from build123d import *


with BuildPart() as part:
    # Sketch2 → Revolve1 (revolve)
    with BuildSketch(Plane.XY, mode=Mode.PRIVATE) as revolve1_sk:
        with BuildLine():
            Line((0, 0), (6.24, 0))
            Line((6.24, 0), (6.24, 48.588483168))
            ThreePointArc((6.24, 48.588483168), (6.146561159, 49.109622023), (5.877885725, 49.565834731))
            ThreePointArc((5.877885725, 49.565834731), (4.874570596, 52.273796489), (5.877885725, 54.981758248))
            ThreePointArc((5.877885725, 54.981758248), (6.146561159, 55.437970955), (6.24, 55.95910981))
            Line((6.24, 55.95910981), (6.24, 55.998530254))
            ThreePointArc((6.24, 55.998530254), (4.278763618, 60.161301491), (0, 61.854610207))
            Line((0, 61.854610207), (0, 0))
        make_face()
    revolve(revolve1_sk.sketch.rotate(Axis((0, 61.854610207, 0), (0, -1, 0)), 180), axis=Axis((0, 61.854610207, 0), (0, -1, 0)))


solid = part.part
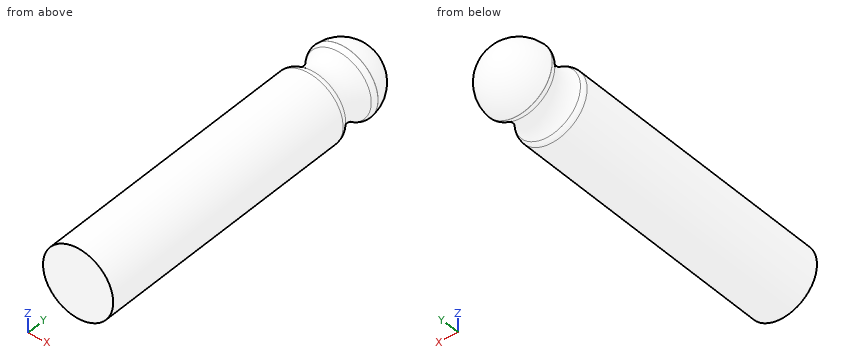
Could you check a few things on this model? Use its own coordinates, in mm. Give positions to 0.01 mm unless a question says otherwise; leave off trailing zeros. Write each loop counter-clockwise with the first axis right and the second up, starting at its lowest first coordinate (ties: lowest second). Pieces come first, ordered by that corner, then holes. Notation, with made-up numbers: (12.25, -16.75) -> (29.25, -16.75) arc R17 ccw to (29.25, -11.75) -> close; hole circle Ø10 at (-9, -28.5). An arc over 180 degrees is marked (long way). Answer as a JSON object with one key per item and string values.
Q1. Suppose I cut it at D-D on y = 51. Write out the boundary of the cut face in (x, z).
Taken from the geometry:
{"outline": "circle Ø10.15 at (0, 0)"}
Q2. Please list where these lines run through material, in increasing order: L1, parallel to X at y = 12.5, z = -0.25; L2, parallel to X at y = 25, z = -2.5; L3, parallel to Y at x = 4.25, z = -0.75.
Taken from the geometry:
{"L1": "x = -6.23 to 6.23", "L2": "x = -5.72 to 5.72", "L3": "y = 0 to 60.13"}
Q3. Suppose I cut it at C-C on y = 30.5. Write out the boundary of the cut face in (x, z).
Taken from the geometry:
{"outline": "circle Ø12.48 at (0, 0)"}
Q4. Will these pins go through, and if not, where does the flat tip stop? pin 1 Ø1.5 at (x, y) = (3, 38.5) entering from +Z; pin 2 Ø4 at (x, y) = (-3, 7) entering from -Z; pin 3 Ø3 at (y, z) = (24.5, 2) entering from +X.
Taken from the geometry:
{"pin 1": "stops at z = 5.82", "pin 2": "stops at z = -6.16", "pin 3": "stops at x = 6.22"}
